The model under review builds one solid part; all positions refer to its coordinate system, in mm. Round coordinates to 2 decimals unless told otherwise and drop trailing zeros. Order: outer loops, then holes, each group sorted by start corner. A loop starts at its lowest first (then second) coordinate and runs counter-clockwise, first axis right, second up. Notation, with made-up numbers: (1.5, 75.25) -> (37.5, 75.25) arc R28 cw to (37.5, 104.25) -> close; hole circle Ø8 at (44, 29). An arc over 180 degrees is marked (long way). Put each result on its own line as item: value. Start each with the question number.
from build123d import *

# Parameters (mm, degrees)
BOSS_EXTRUDE1_DEPTH = 8
CUT_EXTRUDE1_DEPTH  = 17
FILLET1_R           = 1


with BuildPart() as part:
    # Sketch1 → Boss-Extrude1 (new body, symmetric)
    with BuildSketch(Plane.XY):
        Polygon((0, 0), (60, 0), (0, 100), align=None)
    extrude(amount=BOSS_EXTRUDE1_DEPTH, both=True)

    # Sketch2 → Cut-Extrude1 (cut, through all)
    with BuildSketch(Plane.XY.offset(8)):
        Polygon((0, 0), (0, 10), (10, 0), align=None)
    extrude(amount=-CUT_EXTRUDE1_DEPTH, mode=Mode.SUBTRACT)

    # Fillet1
    fillet1_edges = [part.edges().sort_by_distance(p)[0] for p in [
        (30, 50, 8),
        (30, 50, -8),
    ]]
    fillet(fillet1_edges, radius=FILLET1_R)


solid = part.part
Q1. Draft analysis for pull direction X (two halves, no side actions). For faces 1 (the face through (35, 0, 0)), 2 (the face through (0, 56, 0)), 3 (the face through (30.42, 49.3, 0.1)), state which applies: +X half, -X half, draft (parallel to the pull), parting line (faces both ways), or undercut.
Q2. Wall thickness on probe 1 along Y at (x, z) = (7.5, 0.5); probe 2 along Y at (x, z) = (19.5, 5); probe 3 along Z at (x, y) = (34, 43): over which ranges is each line inside the solid? List them lowest first. Write a range as [from, to].
Q3. Clearance check with flat-ended pins moving along their axes: pin 1 Ø4 at (y, z) = (59.5, 4.5) entering from -X; pin 2 Ø2 at (x, z) = (8.5, -1) entering from +Y; pin 3 Ø2 at (x, z) = (9.5, 3) entering from +Y; pin 4 Ø6 at (x, z) = (23, -5.5) entering from +Y. State where each tip first meets the part, or that it passes through.
Q4. Take a section at A-A on z = 1.75. Give the boundary of the cut face in (x, y), and give its area (3 significant figures).
Calculated:
1. face 1: draft
1. face 2: -X half
1. face 3: +X half
2. probe 1: y = [2.5, 87.5]
2. probe 2: y = [0, 67.5]
2. probe 3: z = [-7.56, 7.56]
3. pin 1: stops at x = 0
3. pin 2: stops at y = 87.5
3. pin 3: stops at y = 85.83
3. pin 4: stops at y = 66.67
4. outline: (0, 10) -> (10, 0) -> (60, 0) -> (0, 100) -> close
4. area: 2,950 mm²
